Source: three-view drawing plus pictorial views. Frame: mm from the lowest corner of the part. A direction names the side the tool comes from. Round coordinates to 2 decimals unless told otherwise and drop trailing zeros. Loops run counter-clockwise (first coordinate to the right, second up) from the corner with the lowest first, then second, coordinate; pieces in that order, holes last. Notation, with made-up numbers: M 39.25,82 L 52.25,82 A9 cw 52.25,91 Z; hole C 49.5,87.25 d7. An arc over 180 degrees is marked long. Answer as a JSON object with one key per item and string values.
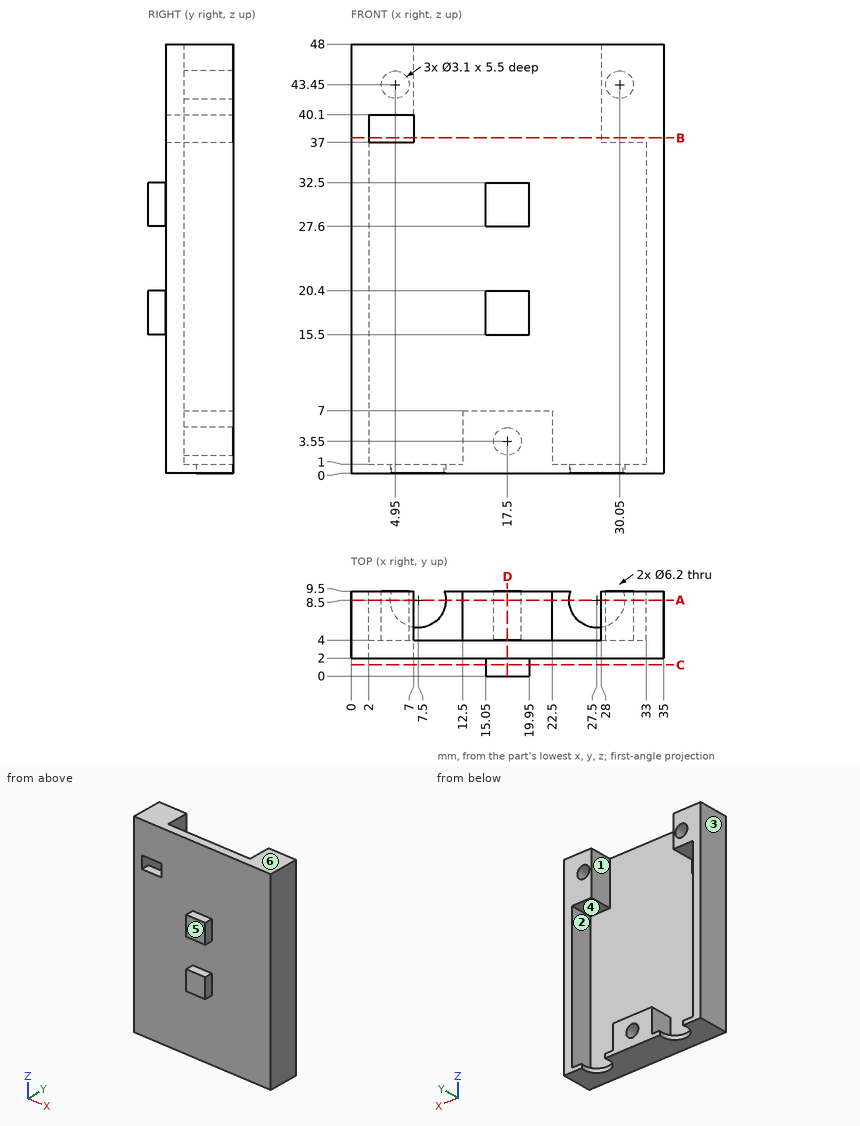
1) Pull-direction query (Z, two-part tool) for the marked faces 4, 5 and 6; classes: +Z half, -Z half, draft (parallel to the pull), parting line (faces both ways), or undercut.
Geometry results:
{"face 4": "undercut", "face 5": "draft", "face 6": "+Z half"}
2) Cut plane D-D on x = 17.5. Return the cut outline in (y, z).
Geometry results:
{"outline": "M 0,15.5 L 2,15.5 L 2,0 L 9.5,0 L 9.5,2 L 4,2 L 4,5.1 L 9.5,5.1 L 9.5,7 L 4,7 L 4,48 L 2,48 L 2,32.5 L 0,32.5 L 0,27.6 L 2,27.6 L 2,20.4 L 0,20.4 Z"}
3) Cut plane A-A on y = 8.5. Return the cut outline in (x, z).
Geometry results:
{"outline": "M 0,0 L 4.4,0 L 4.4,1 L 2,1 L 2,40.1 L 7,40.1 L 7,48 L 0,48 Z; M 10.6,0 L 24.4,0 L 24.4,1 L 22.5,1 L 22.5,7 L 12.5,7 L 12.5,1 L 10.6,1 Z; M 28,37 L 33,37 L 33,1 L 30.6,1 L 30.6,0 L 35,0 L 35,48 L 28,48 Z; hole C 4.95,43.45 d3.1; hole C 17.5,3.55 d3.1; hole C 30.05,43.45 d3.1"}
4) Cut plane C-C on y = 1.25. Return the cut outline in (x, z), and give its area (3 significant figures).
Geometry results:
{"outline": "M 15.05,15.5 L 19.95,15.5 L 19.95,20.4 L 15.05,20.4 Z; M 15.05,27.6 L 19.95,27.6 L 19.95,32.5 L 15.05,32.5 Z", "area": "48.0 mm2"}
5) Cut plane B-B on z = 37.5. Return the cut outline in (x, y).
Geometry results:
{"outline": "M 0,2 L 2,2 L 2,9.5 L 0,9.5 Z; M 7,2 L 35,2 L 35,9.5 L 28,9.5 L 28,4 L 7,4 Z"}
6) First-contact query: pin 1 (1 mm diameter, centred on x = 10.5, z = 37, fed in from +Y); pin 2 (1.6 mm diameter, centred on x = 18.5, y = 1, fed in from +Z); pin 3 (5 mm diameter, centred on x = 28.5, z = 37, fed in from -Y). Flat tips, straight axial feed; report the tip coordinate or a pass-through.
Geometry results:
{"pin 1": "y = 4", "pin 2": "z = 32.5", "pin 3": "y = 2"}
7) Set-up query: the marked faces 1, 2 and 3. Return all of +Z, -Z, +X, -X, +Y, -Y with unobstructed straight access to the full face (end or side cutting, diameter ignored); none if empty.
Geometry results:
{"face 1": "+Z, +Y", "face 2": "+Y", "face 3": "+Z, -Z, -X, +Y, -Y"}
8) Line query: probe 1 along X at (y, z) = (8.5, 0.55); probe 2 along X at (y, z) = (6.4, 43.45); probe 3 along X at (y, z) = (4.5, 17.5). Output: solid intervals per line, ascending.
Geometry results:
{"probe 1": "0 to 4.4, 10.6 to 24.4, 30.6 to 35", "probe 2": "0 to 3.4, 6.5 to 7, 28 to 28.5, 31.6 to 35", "probe 3": "0 to 2, 33 to 35"}
